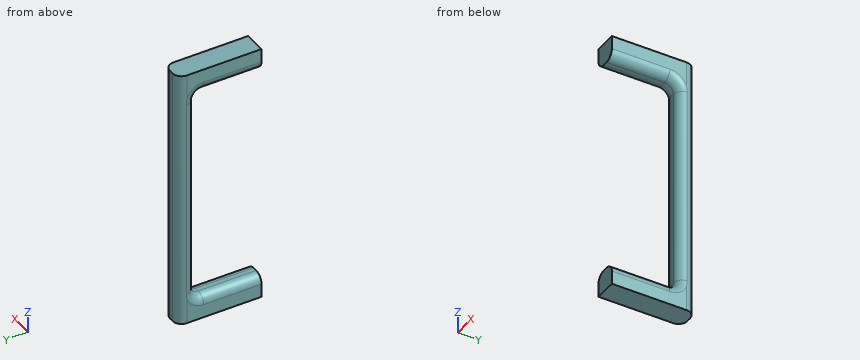
from build123d import *

# Parameters (mm, degrees)
F0_W         = 76.2
F0_H         = 25.4
F1_DEPTH     = 25.4
F2_T1_DEPTH  = 25.4
F2_T3_DEPTH  = 349.25
F2_T5_DEPTH  = 91.44
F2_T7_DEPTH  = 227.33
F2_T10_ANGLE = 90
F2_T12_ANGLE = 90
F2_T14_ANGLE = 90
F2_T16_ANGLE = 90


# Not quite as in the source:
# - a fillet or chamfer that OpenCascade refuses, or shapes differently, is made with other operations: its cross-section is extruded or revolved along the edge and cut away or added


with BuildPart() as f1:
    # F0 (on Right) → F1 (new body)
    with BuildSketch(Plane.YZ):
        Polygon((19.05, 139.6934016338), (0, 139.6934016338), (0, 114.2934016338), (0, 0), (0, -133.3565983662), (-76.2, -133.3565983662), (-76.2, -158.7565983662), (19.05, -158.7565983662), align=None)
        with Locations((-38.1, 126.9934016338)):
            Rectangle(F0_W, F0_H)
    extrude(amount=F1_DEPTH)

    # F2: fillet of radius 10.16 on 10 edges, made by hand

    # F2_s2 → F2_t1 (join)
    with BuildSketch(Plane.YZ):
        with BuildLine():
            ThreePointArc((-10.16, 114.2934016338), (-2.9757951031, 111.3176065306), (0, 104.1334016338))
            Line((0, 104.1334016338), (0, 114.2934016338))
            Line((0, 114.2934016338), (-10.16, 114.2934016338))
        make_face()
        with BuildLine():
            ThreePointArc((0, -123.1965983662), (-2.9757951031, -130.3808032631), (-10.16, -133.3565983662))
            Line((-10.16, -133.3565983662), (0, -133.3565983662))
            Line((0, -133.3565983662), (0, -123.1965983662))
        make_face()
    extrude(amount=F2_T1_DEPTH)

    # F2_s4 → F2_t3 (cut)
    with BuildSketch(Plane.XY.offset(-184.1565983662)):
        with BuildLine():
            ThreePointArc((10.16, 19.05), (2.9757951031, 16.0742048969), (0, 8.89))
            Line((0, 8.89), (0, 19.05))
            Line((0, 19.05), (10.16, 19.05))
        make_face()
        with BuildLine():
            ThreePointArc((15.24, 19.05), (22.4242048969, 16.0742048969), (25.4, 8.89))
            Line((25.4, 8.89), (25.4, 19.05))
            Line((25.4, 19.05), (15.24, 19.05))
        make_face()
    extrude(amount=F2_T3_DEPTH, mode=Mode.SUBTRACT)

    # F2_s6 → F2_t5 (cut)
    with BuildSketch(Plane.XZ.offset(10.16)):
        with BuildLine():
            ThreePointArc((25.4, 124.4534016338), (22.4242048969, 117.2691967369), (15.24, 114.2934016338))
            Line((15.24, 114.2934016338), (25.4, 114.2934016338))
            Line((25.4, 114.2934016338), (25.4, 124.4534016338))
        make_face()
        with BuildLine():
            ThreePointArc((25.4, -143.5165983662), (22.4242048969, -136.3323934694), (15.24, -133.3565983662))
            Line((15.24, -133.3565983662), (25.4, -133.3565983662))
            Line((25.4, -133.3565983662), (25.4, -143.5165983662))
        make_face()
        with BuildLine():
            ThreePointArc((0, -143.5165983662), (2.9757951031, -136.3323934694), (10.16, -133.3565983662))
            Line((10.16, -133.3565983662), (0, -133.3565983662))
            Line((0, -133.3565983662), (0, -143.5165983662))
        make_face()
        with BuildLine():
            ThreePointArc((0, 124.4534016338), (2.9757951031, 117.2691967369), (10.16, 114.2934016338))
            Line((10.16, 114.2934016338), (0, 114.2934016338))
            Line((0, 114.2934016338), (0, 124.4534016338))
        make_face()
    extrude(amount=F2_T5_DEPTH, mode=Mode.SUBTRACT)

    # F2_s8 → F2_t7 (cut)
    with BuildSketch(Plane.XY.offset(-123.1965983662)):
        with BuildLine():
            ThreePointArc((25.4, 10.16), (22.4242048969, 2.9757951031), (15.24, 0))
            Line((15.24, 0), (25.4, 0))
            Line((25.4, 0), (25.4, 10.16))
        make_face()
        with BuildLine():
            ThreePointArc((0, 10.16), (2.9757951031, 2.9757951031), (10.16, 0))
            Line((10.16, 0), (0, 0))
            Line((0, 0), (0, 10.16))
        make_face()
    extrude(amount=F2_T7_DEPTH, mode=Mode.SUBTRACT)

    # F2_s9 → F2_t10 (revolve, cut)
    with BuildSketch(Plane.XZ.offset(10.16)):
        with BuildLine():
            ThreePointArc((0, 124.4534016338), (2.9757951031, 117.2691967369), (10.16, 114.2934016338))
            Line((10.16, 114.2934016338), (0, 114.2934016338))
            Line((0, 114.2934016338), (0, 124.4534016338))
        make_face()
    revolve(axis=Axis((0, -10.16, 104.1334016338), (-1, 0, 0)), revolution_arc=F2_T10_ANGLE, mode=Mode.SUBTRACT)

    # F2_s11 → F2_t12 (revolve, cut)
    with BuildSketch(Plane.XY.offset(-123.1965983662)):
        with BuildLine():
            ThreePointArc((0, 10.16), (2.9757951031, 2.9757951031), (10.16, 0))
            Line((10.16, 0), (0, 0))
            Line((0, 0), (0, 10.16))
        make_face()
    revolve(axis=Axis((0, -10.16, -123.1965983662), (-1, 0, 0)), revolution_arc=F2_T12_ANGLE, mode=Mode.SUBTRACT)

    # F2_s13 → F2_t14 (revolve, cut)
    with BuildSketch(Plane.XY.offset(-123.1965983662)):
        with BuildLine():
            ThreePointArc((25.4, 10.16), (22.4242048969, 2.9757951031), (15.24, 0))
            Line((15.24, 0), (25.4, 0))
            Line((25.4, 0), (25.4, 10.16))
        make_face()
    revolve(axis=Axis((25.4, -10.16, -123.1965983662), (-1, 0, 0)), revolution_arc=F2_T14_ANGLE, mode=Mode.SUBTRACT)

    # F2_s15 → F2_t16 (revolve, cut)
    with BuildSketch(Plane.XZ.offset(10.16)):
        with BuildLine():
            ThreePointArc((25.4, 124.4534016338), (22.4242048969, 117.2691967369), (15.24, 114.2934016338))
            Line((15.24, 114.2934016338), (25.4, 114.2934016338))
            Line((25.4, 114.2934016338), (25.4, 124.4534016338))
        make_face()
    revolve(axis=Axis((25.4, -10.16, 104.1334016338), (-1, 0, 0)), revolution_arc=F2_T16_ANGLE, mode=Mode.SUBTRACT)


solid = f1.part
Part model, mm, in its own coordinate system. Give positions to 0.01 mm unless a question says otherwise; leave off trailing zeros. Loops run counter-clockwise (first coordinate to the right, second up) from the corner with the lowest first, then second, coordinate; pieces in that order, holes last. Notation, with made-up numbers: M 13,-12 L 29,-12 A8 cw 29,-6 Z; hole C 82.25,-3.5 d9. An arc over 180 degrees is marked long. Put each result on its own line as item: value. Start each with the question number.
1) Saw through at A-A (y = -66.5). List the corners of the cut face in (x, z).
2) Flat gauge pins, fed straight in: pin 1 (5.5 mm diameter, centred on x = 13.5, z = 10.5, fed in from -Y); pin 2 (1 mm diameter, centred on x = 5, z = -44, fed in from -Y); pin 3 (1.5 mm diameter, centred on x = 17.5, z = -125, fed in from -Y); pin 4 (6 mm diameter, centred on y = -66.5, z = 109, fed in from -X). Where does each tip first touch, or does it go through?
3) Saw through at B-B (z = 1.5). List the corners of the cut face in (x, y) (3 decimals).
4) Probe probe 1 along Z at (x, y) = (13.25, -66); probe 2 along Z at (x, y) = (4.25, -21); probe 3 along X at (y, z) = (10, 4). List the from-to ranges inside material, lowest first.
Numbers:
1. outline: M 0,-158.76 L 25.4,-158.76 L 25.4,-143.52 A10.16 ccw 15.24,-133.36 L 10.16,-133.36 A10.16 ccw 0,-143.52 Z; M 0,124.45 A10.16 ccw 10.16,114.29 L 15.24,114.29 A10.16 ccw 25.4,124.45 L 25.4,139.69 L 0,139.69 Z
2. pin 1: y = 0
2. pin 2: y = 1.13
2. pin 3: y = -0.12
2. pin 4: through
3. outline: M 0.02,9.525 A10.16 ccw 10.16,0 L 15.24,0 A10.16 ccw 25.38,9.525 A10.16 ccw 15.24,19.05 L 10.16,19.05 A10.16 ccw Z
4. probe 1: -158.76 to -133.36, 114.29 to 139.69
4. probe 2: -158.76 to -135.25, 116.19 to 139.69
4. probe 3: 0.06 to 25.34
